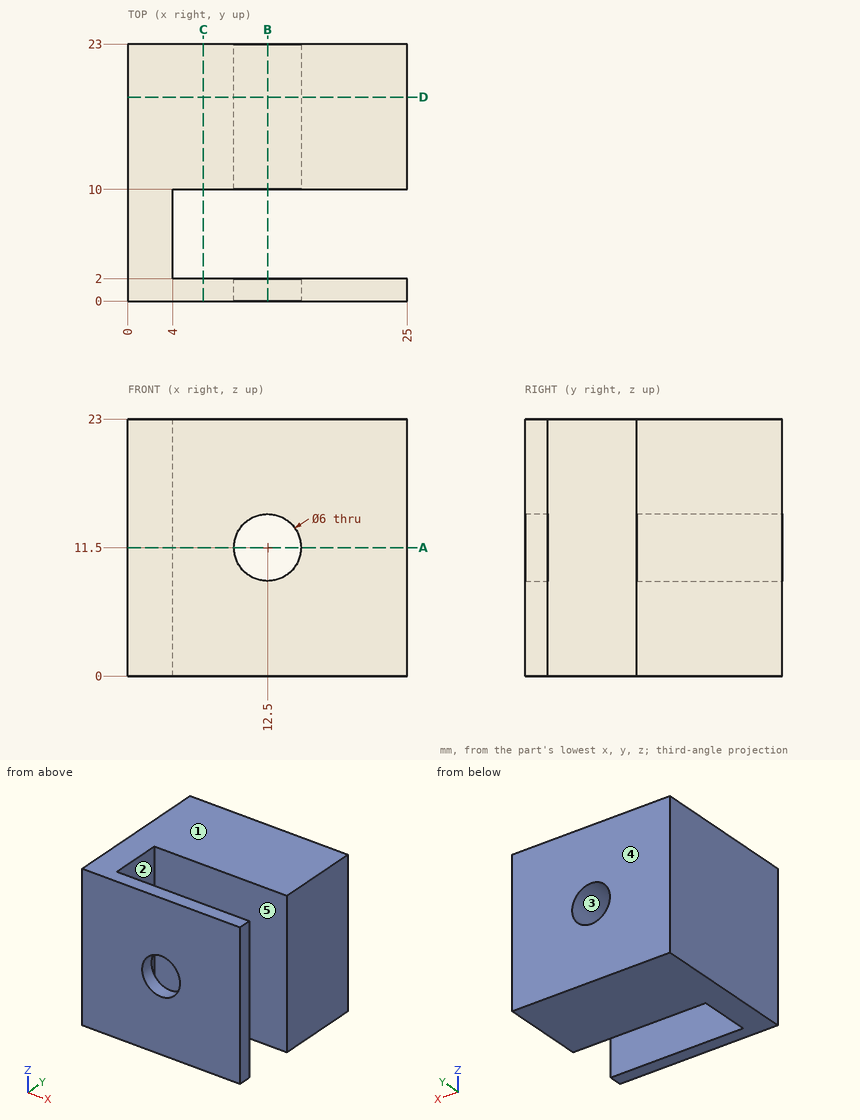
Verification items for this drawing (mm, ordinates from the low corner). A direction names the side the tool comes from. Coordinates: 2 decimals unless noted, no trailing zeros. Write each loop counter-clockwise with the first axis right and the second up, starting at its lowest first coordinate (ties: lowest second). Pieces come first, ordered by that corner, then holes. Notation, with made-up numbers: M 66,55.5 L 113,55.5 A31 ccw 113,94.5 Z; hole C -14,66 d7. An arc over 180 degrees is marked long. Answer as CSV lines item,"result".
Q1. Cross-section at D-D (y = 18.25). Record the boundary of the cut face in (x, z).
Check result:
outline,"M 0,0 L 25,0 L 25,23 L 0,23 Z; hole C 12.5,11.5 d6"
Q2. Cross-section at A-A (z = 11.5). Record the boundary of the cut face in (x, y), then the cut area to 3 significant figures.
Check result:
outline,"M 0,0 L 9.5,0 L 9.5,2 L 4,2 L 4,10 L 9.5,10 L 9.5,23 L 0,23 Z; M 15.5,0 L 25,0 L 25,2 L 15.5,2 Z; M 15.5,10 L 25,10 L 25,23 L 15.5,23 Z"
area,"317 mm^2"
Q3. Cross-section at B-B (x = 12.5). Record the boundary of the cut face in (y, z), then the cut area to 3 significant figures.
Check result:
outline,"M 0,0 L 2,0 L 2,8.5 L 0,8.5 Z; M 0,14.5 L 2,14.5 L 2,23 L 0,23 Z; M 10,0 L 23,0 L 23,8.5 L 10,8.5 Z; M 10,14.5 L 23,14.5 L 23,23 L 10,23 Z"
area,"255 mm^2"
Q4. Mould release check, pull along Z, two halves, no side actions. Record for the marked faces 1, 2 and 3: released by +Z, released by -Z, zero draft, split by the parting line, or undercut.
Check result:
face 1,"released by +Z"
face 2,"zero draft"
face 3,"undercut"
Q5. Set-up check for the marked faces 4 and 5: record each of +Z, -Z, +X, -X, +Y, -Y from which the full face is reachable in a straight line by a thin tool's end or side.
Check result:
face 4,"+Z, -Z, +X, -X, +Y"
face 5,"+Z, -Z, +X"
Q6. Go/stop test with flat-tipped pins: pin 1 (2.5 mm diameter, centred on y = 6, z = 9.5, fed in from +X); pin 2 (3.5 mm diameter, centred on x = 12.5, z = 11.5, fed in from +Y). Record where each tip stops, or that it passes through.
Check result:
pin 1,"x = 4"
pin 2,"through"
Q7. Material ranges on probe 1 along X at (y, z) = (1.3, 11.5); probe 2 along Y at (x, z) = (21.75, 17.25); probe 3 along Z at (x, y) = (12.5, 19.5), recorded low to high. Write a range as from..to.
Check result:
probe 1,"0..9.5, 15.5..25"
probe 2,"0..2, 10..23"
probe 3,"0..8.5, 14.5..23"
Q8. Cross-section at C-C (x = 6.75). Record the boundary of the cut face in (y, z).
Check result:
outline,"M 0,0 L 2,0 L 2,23 L 0,23 Z; M 10,0 L 23,0 L 23,23 L 10,23 Z"
